Part model, mm, in its own coordinate system. Round coordinates to 2 decimals unless told otherwise and drop trailing zeros. Loops run counter-clockwise (first coordinate to the right, second up) from the corner with the lowest first, then second, coordinate; pieces in that order, holes last.
Autodesk Inventor part; units mm, degrees
ref_plane "YZ Plane" through (0, 0, 0) normal (1, 0, 0) x (0, 1, 0)
ref_plane "XZ Plane" through (0, 0, 0) normal (0, 1, 0) x (-1, 0, 0)
ref_plane "XY Plane" through (0, 0, 0) normal (0, 0, 1) x (1, 0, 0)
sketch "스케치1" plane through (0, 0, 0) normal (0, 1, 0) x (-1, 0, 0)
  line L0 (-43, 66) -> (-249, 66)
  line L1 (-249, 66) -> (-249, -209)
  line L2 (-249, -209) -> (-43, -209)
  line L3 (-43, -209) -> (-43, 66)
  point P0 (0, 0)
  dimension "d0" = 206
  dimension "d1" = 275
extrude "돌출1" add sketch "스케치1" along normal blind 2
sketch "스케치2" plane through (0, 2, 0) normal (0, 1, 0) x (1, 0, 0)
  line L0 (43, -66) -> (249, -66)
  line L1 (249, -66) -> (248, -66)
  line L2 (248, -66) -> (248, 209)
  line L3 (249, 209) -> (43, 209)
  line L4 (43, 209) -> (43, -66)
  line L5 (43, -66) -> (44, -66)
  line L6 (44, -66) -> (44, 209)
  line L7 (44, 209) -> (49.4, 209)
  line L8 (49.4, 209) -> (49.4, -66)
  line L9 (248, -66) -> (242.6, -66)
  line L10 (242.6, -66) -> (242.6, 209)
  line L11 (49.4, -66) -> (44, -66)
  line L12 (49.4, 209) -> (44, 209)
  point P0 (0, 0)
  dimension "d4" = 1
  dimension "d5" = 5.4
  dimension "d6" = 5.4
  dimension "d9" = 1
extrude "돌출2" cut sketch "스케치2" against normal blind 1 contours L6 L3 L8 L0 | L10 L3 L2 L0
sketch "스케치3" plane through (0, 2, 0) normal (0, 1, 0) x (1, 0, 0)
  line L0 (197.8, 27.6733) -> (203, 27.6733)
  line L1 (203, 27.6733) -> (203, 51.8733)
  line L2 (203, 51.8733) -> (197.8, 51.8733)
  line L3 (197.8, 51.8733) -> (197.8, 27.6733)
  point P0 (0, 0)
  dimension "d10" = 5.2
  dimension "d11" = 24.2
extrude "돌출3" cut sketch "스케치3" against normal blind 1
sketch "스케치4" plane through (0, 2, 0) normal (0, 1, 0) x (1, 0, 0)
  line L0 (94.2, 171) -> (89, 171)
  line L1 (89, 171) -> (89, 147)
  line L2 (89, 147) -> (94.2, 147)
  line L3 (94.2, 147) -> (94.2, 171)
  point P0 (0, 0)
  dimension "d14" = 5.2
extrude "돌출4" cut sketch "스케치4" against normal blind 1
sketch "스케치5" plane through (0, 0, 0) normal (0, -1, 0) x (1, 0, 0)
  line L0 (43, -209) -> (43, 66)
  line L1 (43, 66) -> (1, 66)
  line L2 (1, 66) -> (1, 21)
  line L3 (1, 21) -> (43, 21)
  line L4 (249, 66) -> (291, 66)
  line L5 (291, 66) -> (291, 21)
  line L6 (291, 21) -> (249, 21)
  line L7 (249, 66) -> (249, -209)
  point P0 (0, 0)
  dimension "d17" = 42
  dimension "d18" = 45
  dimension "d19" = 42
  dimension "d20" = 45
extrude "돌출5" add sketch "스케치5" against normal blind 2
sketch "스케치6" plane through (0, 2, 0) normal (0, 1, 0) x (1, 0, 0)
  line L0 (44, -66) -> (44, 209)
  line L1 (44, 209) -> (43, 209)
  line L2 (43, 209) -> (43, -21)
  line L3 (43, -21) -> (1, -21)
  line L4 (1, -21) -> (1, -66)
  line L5 (1, -66) -> (44, -66)
  line L6 (248, 209) -> (248, -66)
  line L7 (248, -66) -> (291, -66)
  line L8 (291, -66) -> (291, -21)
  line L9 (291, -21) -> (249, -21)
  line L10 (249, -21) -> (249, 209)
  line L11 (249, 209) -> (248, 209)
  line L12 (2, -66) -> (2, -21)
  line L13 (1, -66) -> (291, -66)
  line L14 (7.4, -66) -> (7.4, -21)
  line L15 (248, -66) -> (291, -66)
  line L16 (290, -66) -> (290, -21)
  line L17 (284.6, -66) -> (284.6, -21)
  line L18 (291, -21) -> (249, -21)
  point P0 (0, 0)
  dimension "d23" = 5.4
  dimension "d24" = 1
  dimension "d25" = 1
  dimension "d26" = 5.4
extrude "돌출6" cut sketch "스케치6" against normal blind 1 contours L5 L12 L3 L14 | L17 L9 L16 L7
properties part number "밑판" material "알루미늄 6061"
1) Wall check: line 1 along X through (y, z) = (1.1, -193); line 2 along Z through (x, y) = (202.5, 1.6); line 3 along X through (y, z) = (0.25, -125.5). Give the ranges that are in metal, low to high.
Values:
line 1: x = 43 to 44, 49.4 to 242.6, 248 to 249
line 2: z = -209 to -51.87, -27.67 to 66
line 3: x = 43 to 249
2) Slice it at A-A, the plane y = 1.45. Give the number of separate pieces and of enclosed holes in the cut face, then the cut area to 3 significant figures.
Values:
separate pieces: 5
enclosed holes: 2
area: 56,700 mm2
3) Drop flat-ended pins along their axis: pin 1 Ø0.5 at (y, z) = (1.5, -23) entering from -X; pin 2 Ø1 at (x, y) = (265.5, 0.5) entering from -Z; pin 3 Ø2.5 at (x, z) = (244.5, -10.5) entering from +Y. Give the stop position or say it passes through.
Values:
pin 1: stops at x = 43
pin 2: stops at z = 21
pin 3: stops at y = 1
4) Slice it at B-B, the plane z = -47. Give the cut face in (x, y).
Values:
outline: (43, 0) - (249, 0) - (249, 2) - (248, 2) - (248, 1) - (242.6, 1) - (242.6, 2) - (203, 2) - (203, 1) - (197.8, 1) - (197.8, 2) - (49.4, 2) - (49.4, 1) - (44, 1) - (44, 2) - (43, 2) - close
5) Slice it at C-C, the plane x = 273. Give the cut face in (y, z), then the cut area to 3 significant figures.
Values:
outline: (0, 21) - (2, 21) - (2, 66) - (0, 66) - close
area: 90.0 mm2
6) Slice it at D-D, the plane z = 29. Give the cut face in (x, y).
Values:
outline: (1, 0) - (291, 0) - (291, 2) - (290, 2) - (290, 1) - (284.6, 1) - (284.6, 2) - (248, 2) - (248, 1) - (242.6, 1) - (242.6, 2) - (49.4, 2) - (49.4, 1) - (44, 1) - (44, 2) - (7.4, 2) - (7.4, 1) - (2, 1) - (2, 2) - (1, 2) - close
